Part print with two shaded views. Sizes in mm from the minimum x, y, z corner. Coordinates: 2 decimals unless noted, no trailing zeros. Order: outer loops, then holes, each group sorted by start corner. A loop starts at its lowest first (then second) coordinate and runs counter-clockwise, first axis right, second up.
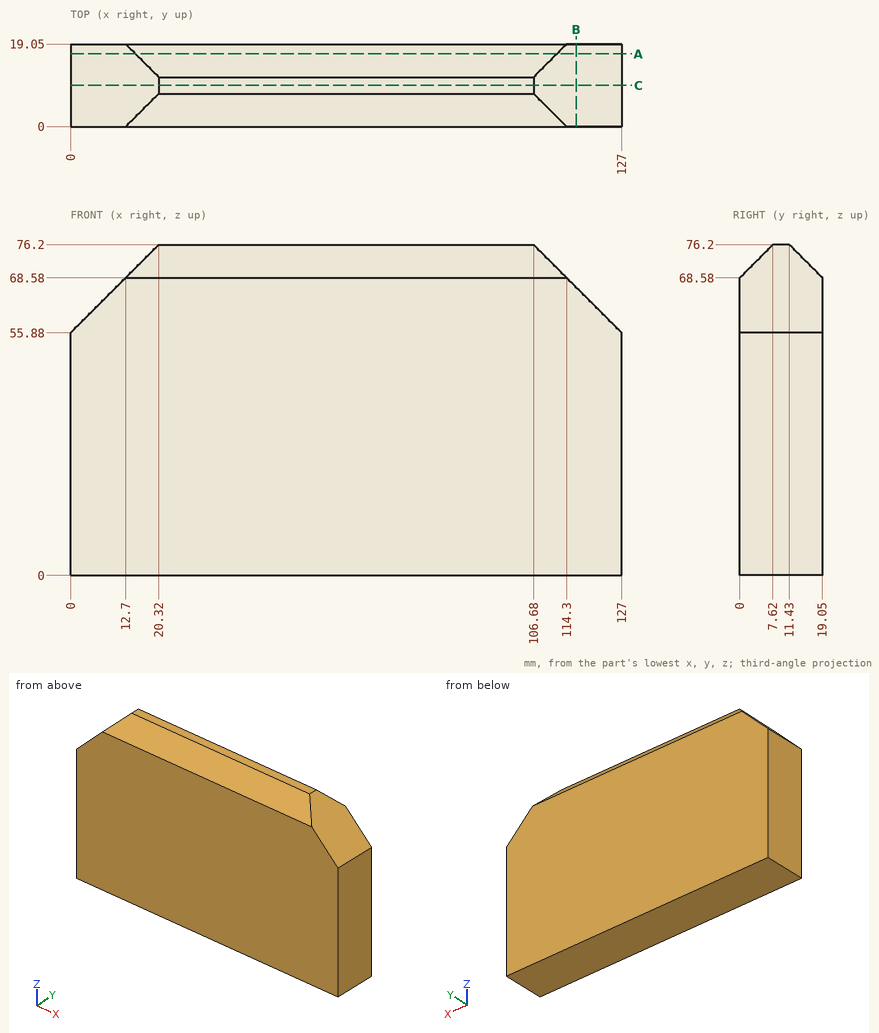
Q1. Cut at B-B on x = 116.5. Write the cut outline in (y, z), and give its area (3 significant figures).
Results list:
outline: (0, 0) - (19.05, 0) - (19.05, 66.38) - (0, 66.38) - close
area: 1,260 mm2
Q2. Cut at C-C on y = 9.5. Write the cut outline in (x, z), and give its area (3 significant figures).
Results list:
outline: (0, 0) - (127, 0) - (127, 55.88) - (106.68, 76.2) - (20.32, 76.2) - (0, 55.88) - close
area: 9,260 mm2
Q3. Wall check: line 1 along Z through (x, y) = (20, 3); line 2 along Z through (x, y) = (99.5, 3.5); line 3 along X through (y, z) = (17.75, 61). Give the ranges that are in metal, low to high.
Results list:
line 1: z = 0 to 71.58
line 2: z = 0 to 72.08
line 3: x = 5.12 to 121.88
Q4. Pin check, flat tip, straight feed: pin 1 Ø3 at (x, y) = (20.5, 4) entering from +Z. Stop position of the tip, or through.
Results list:
pin 1: stops at z = 74.08
Q5. Cut at A-A on y = 16.75. Write the cut outline in (x, z), and give its area (3 significant figures).
Results list:
outline: (0, 0) - (127, 0) - (127, 55.88) - (112, 70.88) - (15, 70.88) - (0, 55.88) - close
area: 8,780 mm2
